Part model, mm, in its own coordinate system. Coordinates: 2 decimals unless noted, no trailing zeros. Order: outer loops, then holes, each group sorted by start corner. A loop starts at its lowest first (then second) coordinate and runs counter-clockwise, first axis right, second up.
1) Cut at C-C (y = -6.5). List the corners of the cut face in (x, z), and give its area (3 significant figures).
2) Wall check: L1, parallel to Y at x = -11, z = 3.5; L2, parallel to Y at x = 149, z = -16. Give the ranges that are in metal, low to high.
3) Pin check, flat tip, straight feed: pin 1 Ø1 at (y, z) = (-5, -17) entering from +X. Stop position of the tip, or through.
```python
from build123d import *

# Parameters (mm, degrees)
F1_DEPTH = 9.525
F2_SIZE2 = 4.7625
F2_SIZE  = 25.4
F3_SIZE2 = 25.39999
F3_SIZE  = 4.76249
F4_SIZE2 = 4.7625
F4_SIZE  = 25.4
F5_SIZE2 = 25.39999
F5_SIZE  = 4.76249


# Not quite as in the source:
# - a fillet or chamfer is up to 0.001 mm smaller than in the source, because OpenCascade refuses the exact size


with BuildPart() as f1:
    # F0 (on Front) → F1 (new body)
    with BuildSketch(Plane.XZ):
        Polygon((112.3986273699, 65.3573278389), (-167.0013726301, -29.8926721611), (163.1986273699, -29.8926721611), (188.5986273699, 65.3573278389), align=None)
    extrude(amount=F1_DEPTH)

    # F2
    f2_edges = [f1.edges().sort_by_distance(p)[0] for p in [
        (-27.301373, -9.525, 17.732328),
    ]]
    f2_side = f1.faces().sort_by_distance((58.423627, -9.525, 7.810453))[0]
    chamfer(f2_edges, length=F2_SIZE, length2=F2_SIZE2, reference=f2_side)

    # F3 (size 4.7625 and 25.4 in the source; OpenCascade refuses exactly that, so slightly less here)
    f3_edges = [f1.edges().sort_by_distance(p)[0] for p in [
        (-27.301373, 0, 17.732328),
    ]]
    f3_side = f1.faces().sort_by_distance((-27.301373, -2.38125, 17.732328))[0]
    chamfer(f3_edges, length=F3_SIZE, length2=F3_SIZE2, reference=f3_side)

    # F4
    f4_edges = [f1.edges().sort_by_distance(p)[0] for p in [
        (175.772766, -9.525, 17.260346),
    ]]
    f4_side = f1.faces().sort_by_distance((87.753798, -9.525, 1.542673))[0]
    chamfer(f4_edges, length=F4_SIZE, length2=F4_SIZE2, reference=f4_side)

    # F5 (size 4.7625 and 25.4 in the source; OpenCascade refuses exactly that, so slightly less here)
    f5_edges = [f1.edges().sort_by_distance(p)[0] for p in [
        (175.772767, 0, 17.260352),
    ]]
    f5_side = f1.faces().sort_by_distance((175.896628, -2.381619, 17.72483))[0]
    chamfer(f5_edges, length=F5_SIZE, length2=F5_SIZE2, reference=f5_side)


solid = f1.part
```
Geometry check:
1. outline: (-138.28, -29.89) - (153.61, -29.89) - (179.01, 65.36) - (141.12, 65.36) - close
1. area: 15,700 mm2
2. L1: y = -8.27 to -1.25
2. L2: y = -8.01 to -1.52
3. pin 1: stops at x = 166.75
